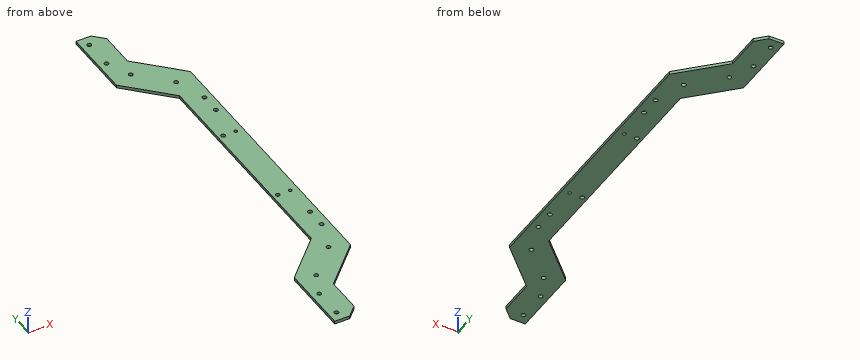
```python
from build123d import *

# Parameters (mm, degrees)
BOSS_EXTRUDE1_DEPTH = 3
BOSS_EXTRUDE2_DEPTH = 3
CHAMFER1_SIZE       = 10
SKETCH3_R           = 2.15
SKETCH3_R_2         = 1.6
CUT_EXTRUDE1_DEPTH  = 10
SKETCH4_R           = 2.15
CUT_EXTRUDE2_DEPTH  = 10


with BuildPart() as part:
    # Sketch1 → Boss-Extrude1 (new body)
    with BuildSketch(Plane.XY):
        Polygon((-372.700177837, -225), (-357.700177837, -225), (-347.700177837, -225), (-347.700177837, -179.142135624), (-307.700177837, -139.142135624), (-307.700177837, -125), (-307.700177837, 125), (-307.700177837, 139.142135624), (-347.700177837, 179.142135624), (-347.700177837, 225), (-357.700177837, 225), (-372.700177837, 225), (-372.700177837, 168.786796564), (-332.700177837, 128.786796564), (-332.700177837, -128.786796564), (-372.700177837, -168.786796564), align=None)
    extrude(amount=BOSS_EXTRUDE1_DEPTH)

    # Sketch2 → Boss-Extrude2 (add)
    with BuildSketch(Plane.XY.offset(3)):
        Polygon((-372.700177837, 168.786796564), (-372.700177837, 154.644660941), (-332.700177837, 114.644660941), (-332.700177837, 128.786796564), align=None)
        Polygon((-372.700177837, -168.786796564), (-372.700177837, -154.644660941), (-332.700177837, -114.644660941), (-332.700177837, -128.786796564), align=None)
    extrude(amount=-BOSS_EXTRUDE2_DEPTH)

    # Chamfer1
    chamfer1_edges = [part.edges().sort_by_distance(p)[0] for p in [
        (-347.700177837, 225, 1.5),
        (-347.700177837, -225, 1.5),
    ]]
    chamfer(chamfer1_edges, length=CHAMFER1_SIZE)

    # Sketch3 → Cut-Extrude1 (cut)
    with BuildSketch(Plane.XY.offset(3)):
        with Locations((-327.700177837, 47.5)):
            Circle(SKETCH3_R)
        with Locations((-315.200177837, 47.5)):
            Circle(SKETCH3_R_2)
        with Locations((-327.700177837, -47.5)):
            Circle(SKETCH3_R)
        with Locations((-315.200177837, -47.5)):
            Circle(SKETCH3_R_2)
    extrude(amount=-CUT_EXTRUDE1_DEPTH, mode=Mode.SUBTRACT)

    # Sketch4 → Cut-Extrude2 (cut)
    with BuildSketch(Plane(origin=(0, 0, 0), x_dir=(-1, 0, 0), z_dir=(0, 0, -1))):
        with Locations((365.200177837, 215)):
            Circle(SKETCH4_R)
        with Locations((365.200177837, 185)):
            Circle(SKETCH4_R)
        with Locations((354.593576119, 161.286796564)):
            Circle(SKETCH4_R)
        with Locations((325.806779555, 132.5)):
            Circle(SKETCH4_R)
        with Locations((315.200177837, 101.893398282)):
            Circle(SKETCH4_R)
        with Locations((315.200177837, 81.893398282)):
            Circle(SKETCH4_R)
        with Locations(Location((315.200177837, -81.893398282, 0), (0, 0, 180))):
            Circle(SKETCH4_R)
        with Locations(Location((315.200177837, -101.893398282, 0), (0, 0, 180))):
            Circle(SKETCH4_R)
        with Locations(Location((325.806779555, -132.5, 0), (0, 0, 180))):
            Circle(SKETCH4_R)
        with Locations(Location((354.593576119, -161.286796564, 0), (0, 0, 180))):
            Circle(SKETCH4_R)
        with Locations(Location((365.200177837, -185, 0), (0, 0, 180))):
            Circle(SKETCH4_R)
        with Locations(Location((365.200177837, -215, 0), (0, 0, 180))):
            Circle(SKETCH4_R)
    extrude(amount=-CUT_EXTRUDE2_DEPTH, mode=Mode.SUBTRACT)


solid = part.part
```
Source: CAD feature listing. Evaluate the final solid. Frame: model axes, mm. Give positions to 0.01 mm unless a question says otherwise; leave off trailing zeros. Loops run counter-clockwise (first coordinate to the right, second up) from the corner with the lowest first, then second, coordinate; pieces in that order, holes last. Notation, with made-up numbers: (34, 3) - (47, 3) arc R22 cw to (47, 23) - close; hole circle Ø6 at (-38, 34.5). An arc over 180 degrees is marked (long way). Use CSV: the item, a comma, the result in double quotes.
1) Cut plane A-A (z = 0.5). Count the separate pieces of the cut face and the enclosed holes in it, and give its area (3 significant figures).
Worked out:
separate pieces,"1"
enclosed holes,"16"
area,"12,900 mm^2"
2) Cut plane B-B (y = 27). Output: boundary loops of the cut face in (x, z).
Worked out:
outline,"(-332.7, 0) - (-307.7, 0) - (-307.7, 3) - (-332.7, 3) - close"
3) Line query: line 1 (Y direction, x = -353, z = 0.4); line 2 (Y direction, x = -355.5, z = 2.05); line 3 (Y direction, x = -338.5, z = 0.75). Output: solid intervals per line, ascending.
Worked out:
line 1,"y = -220.3 to -162.73, -159.84 to -134.94, 134.94 to 159.84, 162.73 to 220.3"
line 2,"y = -222.8 to -163.24, -159.34 to -137.44, 137.44 to 159.34, 163.24 to 222.8"
line 3,"y = -169.94 to -120.44, 120.44 to 169.94"
4) Pin query (flat end, axial travel): P1, Ø2.5, axis at x = -315.2, y = 47.5, coming from the -Z side; P2, Ø1.5, axis at y = -194.5, z = 1, coming from the +X side; P3, Ø1.5, axis at y = 9.5, z = 2, coming from the -X side. Return the tip coordinate at first contact, or that it passes through.
Worked out:
P1,"passes through"
P2,"stops at x = -347.7"
P3,"stops at x = -332.7"
